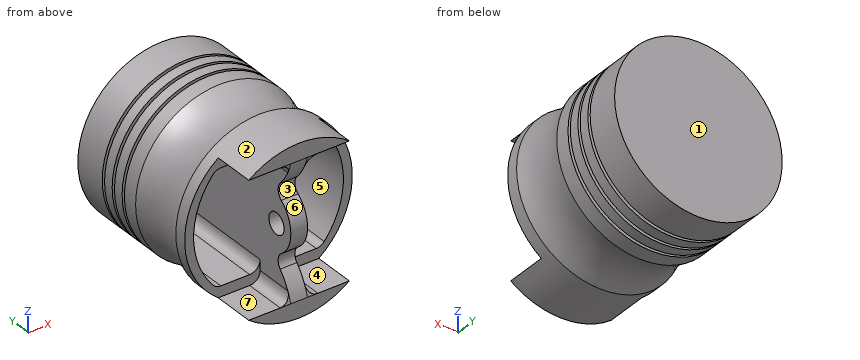
from build123d import *

# Parameters (mm, degrees)
SKETCH2_W                = 40
SKETCH2_H                = 70
SKETCH4_W                = 40
SKETCH4_H                = 20
CUT_EXTRUDE1_DEPTH       = 51
CUT_EXTRUDE1_DEPTH_BACK  = 47
SKETCH5_W                = 64
SKETCH5_H                = 20
BOSS_EXTRUDE1_DEPTH      = 4
BOSS_EXTRUDE1_DEPTH_BACK = 4
SKETCH3_R                = 5
FILLET2_R                = 5
FILLET3_R                = 5
CUT_EXTRUDE2_DEPTH       = 60
SKETCH8_W                = 3
SKETCH8_H                = 1.5


with BuildPart() as part:
    # Sketch2 → Revolve1 (revolve)
    with BuildSketch(Plane(origin=(0, 0, 0), x_dir=(0, 0, -1), z_dir=(1, 0, 0)), mode=Mode.PRIVATE) as revolve1_sk:
        with Locations((20, 91.106067618)):
            Rectangle(SKETCH2_W, SKETCH2_H)
    revolve(revolve1_sk.sketch.rotate(Axis((0, 126.106067618, 0), (0, -1, 0)), 180), axis=Axis((0, 126.106067618, 0), (0, -1, 0)))

    # Sketch4 → Revolve2 (revolve)
    with BuildSketch(Plane(origin=(0, 0, 0), x_dir=(0, 0, -1), z_dir=(1, 0, 0)), mode=Mode.PRIVATE) as revolve2_sk:
        with Locations((20, 46.106067618)):
            Rectangle(SKETCH4_W, SKETCH4_H)
    revolve(revolve2_sk.sketch.rotate(Axis((0, 56.106067618, 0), (0, -1, 0)), 180), axis=Axis((0, 56.106067618, 0), (0, -1, 0)))

    # Sketch5 → Cut-Extrude1 (cut, two sides: drawn at the far end of the back side and taken through both)
    with BuildSketch(Plane(origin=(0, 0, 0), x_dir=(0, 0, -1), z_dir=(1, 0, 0)).offset(-CUT_EXTRUDE1_DEPTH_BACK)):
        with Locations((0, 46.106067618)):
            Rectangle(SKETCH5_W, SKETCH5_H)
    extrude(amount=CUT_EXTRUDE1_DEPTH + CUT_EXTRUDE1_DEPTH_BACK, mode=Mode.SUBTRACT)

    # Sketch3 → Boss-Extrude1 (add, two sides: drawn at the far end of the back side and taken through both)
    with BuildSketch(Plane(origin=(0, 0, 0), x_dir=(0, 0, -1), z_dir=(1, 0, 0)).offset(-BOSS_EXTRUDE1_DEPTH_BACK)):
        with BuildLine():
            Line((-32, 56.106067618), (-14.456832295, 56.106067618))
            Line((-14.456832295, 56.106067618), (14.456832295, 56.106067618))
            Line((14.456832295, 56.106067618), (32, 56.106067618))
            Line((32, 56.106067618), (32, 36.106067618))
            ThreePointArc((32, 36.106067618), (25.399471898, 38.812393939), (19.624541582, 43.00063381))
            ThreePointArc((19.624541582, 43.00063381), (15.729589271, 44.305817394), (12.171473884, 42.25302111))
            ThreePointArc((12.171473884, 42.25302111), (0, 36.019732208), (-12.171473884, 42.25302111))
            ThreePointArc((-12.171473884, 42.25302111), (-15.729589271, 44.305817394), (-19.624541582, 43.00063381))
            ThreePointArc((-19.624541582, 43.00063381), (-25.399471898, 38.812393939), (-32, 36.106067618))
            Line((-32, 36.106067618), (-32, 56.106067618))
        make_face()
        with Locations((0, 45.417119487)):
            Circle(SKETCH3_R, mode=Mode.SUBTRACT)
    extrude(amount=BOSS_EXTRUDE1_DEPTH + BOSS_EXTRUDE1_DEPTH_BACK)

    # Fillet2
    # the kernel refuses this fillet: 5 mm, written as the material it adds along each edge
    with BuildSketch(Plane(origin=(4, 36.106067618, 32), x_dir=(1, 0, 0), z_dir=(0, 1, 0))) as fillet2_piece_1_section:
        with BuildLine():
            CenterArc((FILLET2_R, FILLET2_R), FILLET2_R, 180, 90)
            Line((0, FILLET2_R), (0, 0))
            Line((0, 0), (FILLET2_R, 0))
        make_face()
    fillet2_piece_1 = extrude(amount=32.5, mode=Mode.PRIVATE)
    fillet2_piece_1 = fillet2_piece_1 & Plane(origin=(5.143552766, 65.019732208, 40), x_dir=(0, -0.7339699466021848, -0.6791819472606629), z_dir=(-1, 0, 0)) * Cylinder(30, 85, mode=Mode.PRIVATE)
    add(fillet2_piece_1)

    # Fillet3
    # the kernel refuses this fillet: 5 mm, written as the material it adds along each edge
    with BuildSketch(Plane(origin=(-4, 36.106067618, 32), x_dir=(0, 0, -1), z_dir=(0, 1, 0))) as fillet3_piece_1_section:
        with BuildLine():
            CenterArc((FILLET3_R, FILLET3_R), FILLET3_R, 180, 90)
            Line((0, FILLET3_R), (0, 0))
            Line((0, 0), (FILLET3_R, 0))
        make_face()
    fillet3_piece_1 = extrude(amount=32.5, mode=Mode.PRIVATE)
    fillet3_piece_1 = fillet3_piece_1 & Plane(origin=(-5.143552934, 65.019732208, 40), x_dir=(0, -0.7339699466019316, -0.6791819472609367), z_dir=(-1, 0, 0)) * Cylinder(30, 85, mode=Mode.PRIVATE)
    add(fillet3_piece_1)
    with BuildSketch(Plane(origin=(-4, 68.606067618, -32), x_dir=(0, 0, 1), z_dir=(0, -1, 0))) as fillet3_piece_2_section:
        with BuildLine():
            CenterArc((FILLET3_R, FILLET3_R), FILLET3_R, 180, 90)
            Line((0, FILLET3_R), (0, 0))
            Line((0, 0), (FILLET3_R, 0))
        make_face()
    fillet3_piece_2 = extrude(amount=32.5, mode=Mode.PRIVATE)
    fillet3_piece_2 = fillet3_piece_2 & Plane(origin=(-5.131975571, 65.019732208, -40), x_dir=(0, -0.9637888196533986, 0.26666666666666256), z_dir=(-1, 0, 0)) * Cylinder(30, 85, mode=Mode.PRIVATE)
    add(fillet3_piece_2)
    with BuildSketch(Plane(origin=(4, 68.606067618, -32), x_dir=(0, 0, 1), z_dir=(0, -1, 0))) as fillet3_piece_3_section:
        with BuildLine():
            CenterArc((FILLET3_R, -FILLET3_R), FILLET3_R, 90, 90)
            Line((0, -FILLET3_R), (0, 0))
            Line((0, 0), (FILLET3_R, 0))
        make_face()
    fillet3_piece_3 = extrude(amount=32.5, mode=Mode.PRIVATE)
    fillet3_piece_3 = fillet3_piece_3 & Plane(origin=(5.131975571, 65.019732208, -40), x_dir=(0, -0.9637888196533986, 0.26666666666666256), z_dir=(-1, 0, 0)) * Cylinder(30, 85, mode=Mode.PRIVATE)
    add(fillet3_piece_3)

    # Sketch7 → Cut-Extrude2 (cut)
    with BuildSketch(Plane.XZ.offset(-56.106067618)):
        with BuildLine():
            Line((-4, -22), (-4, 22))
            ThreePointArc((-4, 22), (-5.464466094, 25.535533906), (-9, 27))
            Line((-9, 27), (-22.759731635, 27))
            ThreePointArc((-22.759731635, 27), (-24.875929217, 26.530089159), (-26.594357126, 25.208683117))
            ThreePointArc((-26.594357126, 25.208683117), (-35.75, 0), (-26.594357126, -25.208683117))
            ThreePointArc((-26.594357126, -25.208683117), (-24.875929217, -26.530089159), (-22.759731635, -27))
            Line((-22.759731635, -27), (-9, -27))
            ThreePointArc((-9, -27), (-5.464466094, -25.535533906), (-4, -22))
        make_face()
        with BuildLine():
            Line((9, -27), (22.759731635, -27))
            ThreePointArc((22.759731635, -27), (24.875929217, -26.530089159), (26.594357126, -25.208683117))
            ThreePointArc((26.594357126, -25.208683117), (35.75, 0), (26.594357126, 25.208683117))
            ThreePointArc((26.594357126, 25.208683117), (24.875929217, 26.530089159), (22.759731635, 27))
            Line((22.759731635, 27), (9, 27))
            ThreePointArc((9, 27), (5.464466094, 25.535533906), (4, 22))
            Line((4, 22), (4, -22))
            ThreePointArc((4, -22), (5.464466094, -25.535533906), (9, -27))
        make_face()
    extrude(amount=-CUT_EXTRUDE2_DEPTH, mode=Mode.SUBTRACT)

    # Sketch8 → Cut-Revolve1 (revolve, cut)
    with BuildSketch(Plane(origin=(0, 0, 0), x_dir=(0, 0, -1), z_dir=(1, 0, 0))):
        with Locations((38.5, 109.356067618)):
            Rectangle(SKETCH8_W, SKETCH8_H)
        with Locations((38.5, 102.856067618)):
            Rectangle(SKETCH8_W, SKETCH8_H)
        with BuildLine():
            Line((40, 61.941769102), (40, 88.270366135))
            ThreePointArc((40, 88.270366135), (37.711050715, 75.106067618), (40, 61.941769102))
        make_face()
        with Locations((38.5, 96.356067618)):
            Rectangle(SKETCH8_W, SKETCH8_H)
    revolve(axis=Axis((0, 45.417119487, 0), (0, 1, 0)), mode=Mode.SUBTRACT)


solid = part.part
Verification items for the finished model (mm, model axes). Face numbers are marked on the shaded views. A direction names the side the tool comes from. Coordinates: 2 decimals unless noted, no trailing zeros. Write each loop counter-clockwise with the first axis right and the second up, starting at its lowest first coordinate (ties: lowest second). Pieces come first, ordered by that corner, then holes. Notation, with made-up numbers: (86.25, 3) - (122.25, 3) arc R25 ccw to (122.25, 17) - close; hole circle Ø4 at (10, 78.25). An arc over 180 degrees is marked (long way). Answer as a JSON object with one key per item and string values.
(1) Cross-section at B-B on y = 84.5. Record the cut outline in (x, z).
Report:
{"outline": "circle Ø77.72 at (0, 0); hole (-26.59, -25.21) arc R5 ccw to (-22.76, -27) - (-9, -27) arc R5 ccw to (-4, -22) - (-4, 22) arc R5 ccw to (-9, 27) - (-22.76, 27) arc R5 ccw to (-26.59, 25.21) arc R39.28 ccw to start; hole (4, -22) arc R5 ccw to (9, -27) - (22.76, -27) arc R5 ccw to (26.59, -25.21) arc R39.28 ccw to (26.59, 25.21) arc R5 ccw to (22.76, 27) - (9, 27) arc R5 ccw to (4, 22) - close"}
(2) Cross-section at C-C on y = 119.5. Record the cut outline in (x, z), plus the area to 3 significant figures.
Report:
{"outline": "circle Ø80 at (0, 0)", "area": "5,030 mm^2"}
(3) Thickness scan on line 1 along X through (y, z) = (65.5, -14); line 2 along X through (y, z) = (113, 18); line 3 along Y through (x, z) = (0.75, 0). Record the ranges inside material, lowest first.
Report:
{"line 1": "-36.31 to -33.17, -4 to 4, 33.17 to 36.31", "line 2": "-35.72 to -31.38, -4 to 4, 31.38 to 35.72", "line 3": "36.02 to 40.42, 50.42 to 126.11"}
(4) Tool access check on the marked faces 4, 5, 6 and 7. Record the directions out of +Z, -Z, +X, -X, +Y, -Y that give a thin tool (end or side, any length) a straight path to the whole face; none if there is none.
Report:
{"face 4": "+X, -Y", "face 5": "-Y", "face 6": "+X, -X, -Y", "face 7": "-X, -Y"}
(5) Mould release check, pull along Z, two halves, no side actions. Record for the marked faces 1, 2 and 3: pulls with the +Z half, pulls with the -Z half, needs draft (parallel to the pull), parting line crosses it, or undercut.
Report:
{"face 1": "needs draft", "face 2": "parting line crosses it", "face 3": "undercut"}
(6) Gauge pin test, flat ends, axial feed: pin 1 Ø1.5 at (x, y) = (24.5, 89.5) entering from -Z; pin 2 Ø1.5 at (x, y) = (-22, 103.5) entering from -Z; pin 3 Ø6 at (y, z) = (50, -28.5) entering from +X. Record the tip position at first contact, or that the pin passes through.
Report:
{"pin 1": "z = -32.19", "pin 2": "z = -33.88", "pin 3": "x = 6.82"}
(7) Cross-section at A-A on y = 98.5. Record the cut outline in (x, z), plus the area to 3 significant figures.
Report:
{"outline": "circle Ø80 at (0, 0); hole (-26.59, -25.21) arc R5 ccw to (-22.76, -27) - (-9, -27) arc R5 ccw to (-4, -22) - (-4, 22) arc R5 ccw to (-9, 27) - (-22.76, 27) arc R5 ccw to (-26.59, 25.21) arc R39.28 ccw to start; hole (4, -22) arc R5 ccw to (9, -27) - (22.76, -27) arc R5 ccw to (26.59, -25.21) arc R39.28 ccw to (26.59, 25.21) arc R5 ccw to (22.76, 27) - (9, 27) arc R5 ccw to (4, 22) - close", "area": "1,980 mm^2"}
